Could you check a few things on this model? Use its own coordinates, in mm. A direction names the side the tool comes from. Give positions to 0.01 mm unless a question says otherwise; leave off trailing zeros. Order: outer loops, then holes, each group sorted by start corner. A loop starts at its lowest first (then second) coordinate and runs counter-clockwise, first axis right, second up.
(1) If I drill on probe 1 along Y at (x, z) = (-2, -13.5); probe 2 along X at (y, z) = (15, -58); probe 3 along Z at (x, y) = (13, 19.5), over which ranges is the centre line in solid material (lowest first)?
(2) Imagine slicing it at C-C, the plane x = -15.5. Write out the boundary of the cut face in (y, z) (3 decimals).
(3) On a 3-axis mill with a long thin cutter (end or side, diameter ignored), from which of +Z, -Z, +X, -X, +Y, -Y can I reach the whole of each face in a straight line? I mean faces 4 (the flat face through (0, 14, -60.25)), 5 (the flat face through (-16, 2.5, -59)), 6 (the flat face through (0, 21.15, -30)), 7 (the cylindrical face through (-16.477, -14.605, -58.729)), 8 (the cylindrical face through (-0.3, -23.08, -1.12)). Say none if no direction works.
(4) Imagine slicing it at A-A, the plane y = 19.5. Write out the boundary of the cut face in (x, z), then the cut area to 3 significant figures.
(5) Will these pins go through, and if not, where does the flat tip stop? pin 1 (2 mm diameter, centred on x = 15.5, y = -15.5, fed in from -Z); pin 2 (3 mm diameter, centred on x = -15.5, y = -15.5, fed in from -Z); pin 3 (3.5 mm diameter, centred on x = 15, z = -59, fed in from +Y); pin 4 (2.5 mm diameter, centred on x = -17, z = -58, fed in from -Y).
(6) If we mould it in two halves opening along Y, with no side actions, what happens to faces 1 (the flat face through (21.15, 22, -30)), 2 (the flat face through (16, 2.5, -59)), 3 (the cylindrical face through (-0.3, 23.08, -59.13))? For each: released by +Y, released by -Y, zero draft, split by the parting line, or undercut.
(7) Imagine slicing it at D-D, the plane y = -15.5. Write out the boundary of the cut face in (x, z) (3 decimals), then the cut area to 3 significant figures.
(8) Imagine slicing it at B-B, the plane z = -7. Write out the boundary of the cut face in (x, y), then the cut area to 3 significant figures.
from build123d import *

# Parameters (mm, degrees)
SM_START               = -21.15
SM_BASE_FLANGE_2_DEPTH = 42.3
SKETCH_11_R            = 1.325
SKETCH_11_R_2          = 11
CUT_EXTRUDE_1_DEPTH    = 66.636175239


# Sheet-metal steps are written as plain solids
with BuildPart() as part:
    # Эскиз6 → Базовая кромка2 (new body)
    with BuildSketch(Plane(origin=(0, 0, 0), x_dir=(0, 0, -1), z_dir=(1, 0, 0)).offset(SM_START)):
        with BuildLine():
            Line((57.25, 2.5), (57.25, 20.41))
            ThreePointArc((57.25, 20.41), (57.033259018, 20.933259018), (56.51, 21.15))
            Line((56.51, 21.15), (3.74, 21.15))
            ThreePointArc((3.74, 21.15), (3.216740982, 20.933259018), (3, 20.41))
            Line((3, 20.41), (3, -20.41))
            ThreePointArc((3, -20.41), (3.216740982, -20.933259018), (3.74, -21.15))
            Line((3.74, -21.15), (56.51, -21.15))
            ThreePointArc((56.51, -21.15), (57.033259018, -20.933259018), (57.25, -20.41))
            Line((57.25, -20.41), (57.25, -2.5))
            Line((57.25, -2.5), (60.25, -2.5))
            Line((60.25, -2.5), (60.25, -20.41))
            ThreePointArc((60.25, -20.41), (59.154579362, -23.054579362), (56.51, -24.15))
            Line((56.51, -24.15), (3.74, -24.15))
            ThreePointArc((3.74, -24.15), (1.095420638, -23.054579362), (0, -20.41))
            Line((0, -20.41), (0, 20.41))
            ThreePointArc((0, 20.41), (1.095420638, 23.054579362), (3.74, 24.15))
            Line((3.74, 24.15), (56.51, 24.15))
            ThreePointArc((56.51, 24.15), (59.154579362, 23.054579362), (60.25, 20.41))
            Line((60.25, 20.41), (60.25, 2.5))
            Line((60.25, 2.5), (57.25, 2.5))
        make_face()
    extrude(amount=SM_BASE_FLANGE_2_DEPTH)

    # Эскиз11 → Вырез-Вытянуть1 (cut, through all)
    with BuildSketch(Plane.XY.offset(-57.25)):
        with Locations((-15.5, 15.5)):
            Circle(SKETCH_11_R)
        with Locations((15.5, 15.5)):
            Circle(SKETCH_11_R)
        with Locations((15.5, -15.5)):
            Circle(SKETCH_11_R)
        Circle(SKETCH_11_R_2)
        with Locations((-15.5, -15.5)):
            Circle(SKETCH_11_R)
    extrude(amount=-CUT_EXTRUDE_1_DEPTH, mode=Mode.SUBTRACT)


solid = part.part
Answer block:
1. probe 1: y = -24.15 to -21.15, 21.15 to 24.15
1. probe 2: x = -21.15 to -16.73, -14.27 to 14.27, 16.73 to 21.15
1. probe 3: z = -60.25 to -57.25, -3 to 0
2. outline: (-24.15, -56.51) arc R3.74 ccw to (-20.41, -60.25) - (-16.825, -60.25) - (-16.825, -57.25) - (-20.41, -57.25) arc R0.74 cw to (-21.15, -56.51) - (-21.15, -3.74) arc R0.74 cw to (-20.41, -3) - (20.41, -3) arc R0.74 cw to (21.15, -3.74) - (21.15, -56.51) arc R0.74 cw to (20.41, -57.25) - (16.825, -57.25) - (16.825, -60.25) - (20.41, -60.25) arc R3.74 ccw to (24.15, -56.51) - (24.15, -3.74) arc R3.74 ccw to (20.41, 0) - (-20.41, 0) arc R3.74 ccw to (-24.15, -3.74) - close; (-14.175, -60.25) - (-2.5, -60.25) - (-2.5, -57.25) - (-14.175, -57.25) - close; (2.5, -60.25) - (14.175, -60.25) - (14.175, -57.25) - (2.5, -57.25) - close
3. face 4: -Z, +X, -X, +Y, -Y
3. face 5: -Z, +X, -X
3. face 6: +X, -X
3. face 7: -Z
3. face 8: +Z, +X, -X, -Y
4. outline: (-21.15, -60.25) - (21.15, -60.25) - (21.15, -57.25) - (-21.15, -57.25) - close; (-21.15, -3) - (21.15, -3) - (21.15, 0) - (-21.15, 0) - close
4. area: 254 mm2
5. pin 1: stops at z = -3
5. pin 2: stops at z = -60.25
5. pin 3: stops at y = 24.08
5. pin 4: stops at y = -24.14
6. face 1: zero draft
6. face 2: undercut
6. face 3: released by +Y
7. outline: (-21.15, -60.25) - (-16.825, -60.25) - (-16.825, -57.25) - (-21.15, -57.25) - close; (-21.15, -3) - (21.15, -3) - (21.15, 0) - (-21.15, 0) - close; (-14.175, -60.25) - (14.175, -60.25) - (14.175, -57.25) - (-14.175, -57.25) - close; (16.825, -60.25) - (21.15, -60.25) - (21.15, -57.25) - (16.825, -57.25) - close
7. area: 238 mm2
8. outline: (-21.15, -24.15) - (21.15, -24.15) - (21.15, -21.15) - (-21.15, -21.15) - close; (-21.15, 21.15) - (21.15, 21.15) - (21.15, 24.15) - (-21.15, 24.15) - close
8. area: 254 mm2
